Could you check a few things on this model? Use its own coordinates, in mm. A direction names the side the tool comes from. Round coordinates to 2 decimals unless told otherwise and drop trailing zeros. Write each loop counter-clockwise with the first axis right and the second up, starting at its lowest first coordinate (ties: lowest second). Pieces come first, ordered by that corner, then holes. Notation, with made-up numbers: (83, 1.5) -> (121, 1.5) arc R33 cw to (121, 33.5) -> close; hole circle Ø2 at (6.5, 61.25). An arc over 180 degrees is marked (long way). Answer in a Markdown table with one row per item.
Autodesk Inventor part; units mm, degrees
ref_plane "YZ Plane" through (0, 0, 0) normal (1, 0, 0) x (0, 1, 0)
ref_plane "XZ Plane" through (0, 0, 0) normal (0, 1, 0) x (-1, 0, 0)
ref_plane "XY Plane" through (0, 0, 0) normal (0, 0, 1) x (1, 0, 0)
sketch "Skizze1" plane through (0, 0, 0) normal (0, 1, 0) x (-1, 0, 0)
  line L0 (22.6442, -7.5) -> (-7.3558, -7.5)
  line L1 (-7.3558, -7.5) -> (-7.3558, -22.5)
  line L2 (-7.3558, -22.5) -> (22.6442, -22.5)
  line L3 (22.6442, -22.5) -> (22.6442, -7.5)
  point P0 (0, 0)
  dimension "d0" = 15
  dimension "d1" = 30
extrude "Extrusion1" add sketch "Skizze1" along normal blind 10
sketch "Skizze2" plane through (0, 10, 0) normal (0, 1, 0) x (1, 0, 0)
  circle A0 centre (-17.6442, 15) radius 3.2574
  circle A1 centre (2.3558, 15) radius 3.4818
  line L0 (-22.6442, 22.5) -> (-22.6442, 7.5)
  line L1 (7.3558, 7.5) -> (7.3558, 22.5)
  line L2 (7.3558, 22.5) -> (-22.6442, 22.5)
  point P0 (0, 0)
  dimension "d4" = 5
  dimension "d5" = 5
  dimension "d6" = 7.5
  dimension "d7" = 7.5
extrude "Extrusion2" add sketch "Skizze2" along normal blind 5
fillet "Rundung1" radius 2 2 edges at (-20.9017, 15, -15) (-1.1261, 15, -15)
properties part number "IR-Sensor"
1) Thinking about a two-plate mould opening in X: for faces 1 (the face through (-18, 15, -15)), 2 (the face through (-7, 10, -15)), 3 (the face through (-22.644, 5, -15)), 4 (the face through (7.356, 5, -15)), which applies, +X half, -X half, draft (parallel to the pull), parting line (faces both ways), or undercut?
Findings:
| item | result |
|---|---|
| face 1 | draft |
| face 2 | undercut |
| face 3 | -X half |
| face 4 | +X half |
2) For faces 5 (the face through (1.6, 11.5, -18.4)), 6 (the face through (2, 15, -15)), which set-ups out of +Z, -Z, +X, -X, +Y, -Y let a thin tool reach every point of the face, with its end or its side?
Findings:
| item | result |
|---|---|
| face 5 | +Y |
| face 6 | +Z, -Z, +X, -X, +Y |
3) Please list where these lines run through material, in increasing order: line 1 (Y direction, x = -16, z = -8.25); line 2 (Z direction, x = 5.5, y = 12.75); line 3 (Z direction, x = -19, y = 14.25).
Findings:
| item | result |
|---|---|
| line 1 | y = 0 to 10 |
| line 2 | z = -16.5 to -13.5 |
| line 3 | z = -17.47 to -12.53 |
4) For pin 1 (7.5 mm diameter, centred on x = -4, z = -17, fed in from +Y), with a flat end and sliding along its axis, tell me the tip position at first contact or that it passes through.
Findings:
| item | result |
|---|---|
| pin 1 | stops at y = 14.4 |
5) Imagine slicing it at A-A, the plane x = -4.5. Please give me the cut outline in (y, z), plus the area to 3 significant figures.
Findings:
| item | result |
|---|---|
| outline | (0, -22.5) -> (10, -22.5) -> (10, -7.5) -> (0, -7.5) -> close |
| area | 150 mm^2 |
6) Imagine slicing it at B-B, the plane z = -20.25. Please give me the cut outline in (x, y).
Findings:
| item | result |
|---|---|
| outline | (-22.64, 0) -> (7.36, 0) -> (7.36, 10) -> (-22.64, 10) -> close |
